Geometry: final body of the model. Coordinates: model frame, mm. A direction names the side the tool comes from. Give positions to 0.01 mm unless a question says otherwise; leave off trailing zeros. Write each loop counter-clockwise with the first axis right and the second up, starting at its lowest first coordinate (ties: lowest second). Pieces come first, ordered by that corner, then holes.
Q1. Cut plane C-C on y = -18. Return the cut outline in (x, z).
Q2. Cut plane A-A on z = 5. Return the cut outline in (x, y), plus the area to 3 significant figures.
Q3. Reachability of faces 1 (the face through (44, -18, 12)), 2 (the face through (-57, 0, 9)), 3 (the face through (44, -10, 0)) from +Z, -Z, +X, -X, +Y, -Y: full face, straight path, thin tool, end or side. Return the list, or none.
Q4. Line query: L1, parallel to Y at x = 33.5, z = 1.5; L2, parallel to X at y = 9.5, z = 17.5; L3, parallel to Z at x = 13.5, y = 5.5. Output: solid intervals per line, ascending.
Q5. Pin query (flat end, axial travel): pin 1 (4 mm diameter, centred on x = 25.5, y = -17.5, fed in from -Z). Return the tip coordinate at first contact, or that it passes through.
Q6. Cut plane D-D on x = 26. Return the cut outline in (y, z).
Q7. Draft query along Y for faces 4 (the face through (-23, -28, 0)), 5 (the face through (44, 13.6, 11)), 6 (the face through (-8, -29.5, 10)). Return one class per face: pulls with the +Y half, pulls with the -Y half, needs draft (parallel to the pull), parting line crosses it, or undercut.
Q8. Cut plane B-B on z = 13. Return the cut outline in (x, y).
```python
from build123d import *

# Parameters (mm, degrees)
SKETCH_W        = 104
SKETCH_H        = 59
PAD_DEPTH       = 20
SKETCH002_W     = 100
SKETCH002_H     = 55
POCKET_DEPTH    = 18
SKETCH003_W     = 5
SKETCH003_H     = 2
PAD001_DEPTH    = 1
SKETCH004_W     = 5
SKETCH004_H     = 2
PAD002_DEPTH    = 1
POCKET001_DEPTH = 2
FILLET_R        = 0.5
FILLET001_R     = 0.4
FILLET002_R     = 0.5
FILLET003_R     = 0.5


with BuildPart() as part:
    # Sketch → Pad (new body)
    with BuildSketch(Plane.XY):
        with Locations((-7, 0)):
            Rectangle(SKETCH_W, SKETCH_H)
    extrude(amount=PAD_DEPTH)

    # Sketch002 (on Face5 of Pad) → Pocket (cut)
    with BuildSketch(Plane(origin=(0, 0, 0), x_dir=(1, 0, 0), z_dir=(0, 0, -1))):
        with Locations((-7, 0)):
            Rectangle(SKETCH002_W, SKETCH002_H)
    extrude(amount=-POCKET_DEPTH, mode=Mode.SUBTRACT)

    # Sketch003 (on Face8 of Pocket) → Pad001 (join)
    with BuildSketch(Plane.XZ.offset(-27.5)):
        with Locations((-18.5, 3)):
            Rectangle(SKETCH003_W, SKETCH003_H)
        with Locations((18.5, 3)):
            Rectangle(SKETCH003_W, SKETCH003_H)
    extrude(amount=PAD001_DEPTH)

    # Sketch004 (on Face10 of Pad001) → Pad002 (join)
    with BuildSketch(Plane(origin=(0, -27.5, 0), x_dir=(-1, 0, 0), z_dir=(0, 1, 0))):
        with Locations((-18.5, 3)):
            Rectangle(SKETCH004_W, SKETCH004_H)
        with Locations((18.5, 3)):
            Rectangle(SKETCH004_W, SKETCH004_H)
    extrude(amount=PAD002_DEPTH)

    # Sketch005 (on Face3 of Pad002) → Pocket001 (cut)
    with BuildSketch(Plane.YZ.offset(45)):
        with BuildLine():
            ThreePointArc((-21.5, 0), (-18, -3.5), (-14.5, 0))
            Line((-14.5, 0), (-14.5, 8.5))
            ThreePointArc((-14.5, 8.5), (-18, 12), (-21.5, 8.5))
            Line((-21.5, 0), (-21.5, 8.5))
        make_face()
        with BuildLine():
            ThreePointArc((-5, 0), (-2.5, -2.5), (0, 0))
            Line((0, 0), (0, 8.5))
            ThreePointArc((0, 8.5), (-2.5, 11), (-5, 8.5))
            Line((-5, 0), (-5, 8.5))
        make_face()
        with BuildLine():
            ThreePointArc((3, 0), (5.5, -2.5), (8, 0))
            Line((8, 0), (8, 8.5))
            ThreePointArc((8, 8.5), (5.5, 11), (3, 8.5))
            Line((3, 0), (3, 8.5))
        make_face()
        with BuildLine():
            ThreePointArc((11, 0), (13.5, -2.5), (16, 0))
            Line((16, 0), (16, 8.5))
            ThreePointArc((16, 8.5), (13.5, 11), (11, 8.5))
            Line((11, 0), (11, 8.5))
        make_face()
    extrude(amount=-POCKET001_DEPTH, mode=Mode.SUBTRACT)

    # Fillet
    fillet_edges = [part.edges().sort_by_distance(p)[0] for p in [
        (-7, 29.5, 20),
        (-59, 0, 20),
        (-7, -29.5, 20),
        (45, 0, 20),
    ]]
    fillet(fillet_edges, radius=FILLET_R)

    # Fillet001
    fillet001_edges = [part.edges().sort_by_distance(p)[0] for p in [
        (45, 29.5, 9.75),
        (45, -29.5, 9.75),
        (-59, 29.5, 9.75),
        (-59, -29.5, 9.75),
    ]]
    fillet(fillet001_edges, radius=FILLET001_R)

    # Fillet002
    fillet002_edges = [part.edges().sort_by_distance(p)[0] for p in [
        (-18.5, -26.5, 2),
        (-21, -26.5, 3),
        (-18.5, -26.5, 4),
        (-16, -26.5, 3),
        (16, -26.5, 3),
        (18.5, -26.5, 2),
        (21, -26.5, 3),
        (18.5, -26.5, 4),
    ]]
    fillet(fillet002_edges, radius=FILLET002_R)

    # Fillet003
    fillet003_edges = [part.edges().sort_by_distance(p)[0] for p in [
        (-21, 26.5, 3),
        (-18.5, 26.5, 4),
        (-18.5, 26.5, 2),
        (-16, 26.5, 3),
        (18.5, 26.5, 2),
        (16, 26.5, 3),
        (18.5, 26.5, 4),
        (21, 26.5, 3),
    ]]
    fillet(fillet003_edges, radius=FILLET003_R)


solid = part.part
```
Data:
1. outline: (-59, 0) - (-57, 0) - (-57, 18) - (43, 18) - (43, 12) - (45, 12) - (45, 19.5) arc R0.5 ccw to (44.5, 20) - (-58.5, 20) arc R0.5 ccw to (-59, 19.5) - close
2. outline: (-59, -29.1) arc R0.4 ccw to (-58.6, -29.5) - (44.6, -29.5) arc R0.4 ccw to (45, -29.1) - (45, -21.5) - (43, -21.5) - (43, -27.5) - (-57, -27.5) - (-57, 27.5) - (43, 27.5) - (43, 16) - (45, 16) - (45, 29.1) arc R0.4 ccw to (44.6, 29.5) - (-58.6, 29.5) arc R0.4 ccw to (-59, 29.1) - close; (43, -14.5) - (45, -14.5) - (45, -5) - (43, -5) - close; (43, 0) - (45, 0) - (45, 3) - (43, 3) - close; (43, 8) - (45, 8) - (45, 11) - (43, 11) - close
2. area: 592 mm2
3. face 1: -Z, +X
3. face 2: -Z
3. face 3: -Z, +X, -X, +Y, -Y
4. L1: y = -29.5 to -27.5, 27.5 to 29.5
4. L2: x = -59 to -57, 43 to 45
4. L3: z = 18 to 20
5. pin 1: stops at z = 18
6. outline: (-29.5, 0) - (-27.5, 0) - (-27.5, 18) - (27.5, 18) - (27.5, 0) - (29.5, 0) - (29.5, 19.5) arc R0.5 ccw to (29, 20) - (-29, 20) arc R0.5 ccw to (-29.5, 19.5) - close
7. face 4: needs draft
7. face 5: undercut
7. face 6: pulls with the -Y half
8. outline: (-59, -29.1) arc R0.4 ccw to (-58.6, -29.5) - (44.6, -29.5) arc R0.4 ccw to (45, -29.1) - (45, 29.1) arc R0.4 ccw to (44.6, 29.5) - (-58.6, 29.5) arc R0.4 ccw to (-59, 29.1) - close; hole (-57, -27.5) - (43, -27.5) - (43, 27.5) - (-57, 27.5) - close
